Check sheet for the modelled part. Datum: model origin and axes. Units: mm. A direction names the side the tool comes from. Coordinates: 2 decimals unless noted, no trailing zeros. Write each loop counter-clockwise with the first axis right and the second up, starting at its lowest first coordinate (ties: lowest second). Pieces come first, ordered by that corner, then holes. Notation, with made-up numbers: (-37, 62) -> (-10, 62) arc R8 ccw to (-10, 71) -> close; hole circle Ø8 at (25.25, -26). An arc over 180 degrees is marked (long way). One line per item, written item: value. Start each with the question number.
1) Set-up check for faces 4 (the cylindrical face through (23.706, -22.68, 3.479)), 5 (the flat face through (13.895, 27, 1)), 6 (the flat face through (-25, 0, 1)), 7 (the flat face through (19, -25, 1)), 8 (the flat face through (-13.895, 27, 1)): record each of +Z, -Z, +X, -X, +Y, -Y from which the full face is reachable in a straight line by a thin tool's end or side.
2) Sectioned sample at B-B on y = 0. Enter the section's corners in (x, z), plus the area to 3 significant figures.
3) Scan lines: line 1 along Y through (x, z) = (0, 0.6); line 2 along Z through (x, y) = (-13, 29); line 3 along X through (y, z) = (23, 1.75). Record each from-to range of solid material in increasing order. Write a range as [from, to].
4) Gauge pin test, flat ends, axial feed: P1, Ø2, axis at x = -17.5, z = 0.5, coming from the +Y side; P2, Ø1, axis at x = 20, z = 1.5, coming from the -Y side; P3, Ø8, axis at x = -9, y = 23.5, coming from the +Z side. Record the tip position at first contact, or that the pin passes through.
5) Sectioned sample at C-C on z = 11.25. Enter the section's corners in (x, y), plus the area to 3 significant figures.
6) Sectioned sample at D-D on x = -16. Enter the section's corners in (y, z).
7) Sectioned sample at A-A on x = 0. Enter the section's corners in (y, z), plus the area to 3 significant figures.
8) Draft check along Y on faces 1 (the cylindrical face through (13.04, 31.6, 0.99)), 2 (the flat face through (-20, -25, 1)), 3 (the cylindrical face through (-21.836, -20.65, 2.535)). Enter one of: +Y half, -Y half, draft (parallel to the pull), parting line (faces both ways), or undercut.
```python
from build123d import *

# Parameters (mm, degrees)
F0_W      = 50
F0_H      = 50
F1_DEPTH  = 2
F2_R      = 2
F3_DEPTH  = 3
F4_R      = 1.5
F5_DEPTH  = 3
F7_DEPTH  = 2
F8_R      = 1.5
F9_DEPTH  = 25
F10_R     = 7.5
F11_DEPTH = 10
F12_R     = 5
F13_DEPTH = 10
F14_DEPTH = 7.7


# Not quite as in the source:
# - a pattern or mirror of a feature is missing from the dataset's text; its kind, count and spacing are read off the source's solid
# - a feature names something its author has since deleted; it is built from what else it names


with BuildPart() as f1:
    # F0 (on Top) → F1 (new body)
    with BuildSketch(Plane.XY):
        Rectangle(F0_W, F0_H)
    extrude(amount=F1_DEPTH)

    # F2 (on face) → F3 (join)
    with BuildSketch(Plane.XY.offset(2)):
        with Locations((-22.6419584364, -21.9144617685)):
            Circle(F2_R)
        with Locations((21.8580415636, -21.9144617685)):
            Circle(F2_R)
        with Locations((21.8580415636, 22.5855382315)):
            Circle(F2_R)
    f3 = extrude(amount=F3_DEPTH)

    # F3_copies: F3 across plane
    add(f3.mirror(Plane.ZX.offset(0.335538)))

    # F4 (on face) → F5 (cut)
    with BuildSketch(Plane.XY.offset(5)):
        with Locations((-22.6419584364, 22.5855382315)):
            Circle(F4_R)
        with Locations((21.8580415636, -21.9144617685)):
            Circle(F4_R)
        with Locations((21.8580415636, 22.5855382315)):
            Circle(F4_R)
        with Locations((-22.6419584364, -21.9144617685)):
            Circle(F4_R)
    extrude(amount=-F5_DEPTH, mode=Mode.SUBTRACT)

    # F6 (on Top) → F7 (join)
    with BuildSketch(Plane.XY):
        with BuildLine():
            ThreePointArc((13.8950906601, 29.5), (13.0164110037, 31.6213203436), (10.8950906601, 32.5))
            Line((10.8950906601, 32.5), (-10.8950906601, 32.5))
            ThreePointArc((-10.8950906601, 32.5), (-13.0164110037, 31.6213203436), (-13.8950906601, 29.5))
            Line((-13.8950906601, 29.5), (-13.8950906601, 25))
            Line((-13.8950906601, 25), (13.8950906601, 25))
            Line((13.8950906601, 25), (13.8950906601, 29.5))
        make_face()
        with BuildLine():
            Line((13.8950906601, -25), (-13.8950906601, -25))
            Line((-13.8950906601, -25), (-13.8950906601, -29.5))
            ThreePointArc((-13.8950906601, -29.5), (-13.0164110037, -31.6213203436), (-10.8950906601, -32.5))
            Line((-10.8950906601, -32.5), (10.8950906601, -32.5))
            ThreePointArc((10.8950906601, -32.5), (13.0164110037, -31.6213203436), (13.8950906601, -29.5))
            Line((13.8950906601, -29.5), (13.8950906601, -25))
        make_face()
    extrude(amount=F7_DEPTH)

    # F8 (on face) → F9 (cut)
    with BuildSketch(Plane.XY.offset(2)):
        with Locations((0, 29.5)):
            Circle(F8_R)
        with Locations((0, -29.5)):
            Circle(F8_R)
    extrude(amount=-F9_DEPTH, mode=Mode.SUBTRACT)

    # F10 (on face) → F11 (join)
    with BuildSketch(Plane.XY.offset(2)):
        Circle(F10_R)
    extrude(amount=F11_DEPTH)

    # F12 (on face) → F13 (cut)
    with BuildSketch(Plane.XY.offset(12)):
        Circle(F12_R)
    extrude(amount=-F13_DEPTH, mode=Mode.SUBTRACT)

    # F14 (cut): faces of the model
    f14_faces = [f1.faces().sort_by_distance(p)[0] for p in [
        (-22.6419584364, -21.9144617685, 2),
        (-22.6419584364, 22.5855382315, 2),
        (21.8580415636, 22.5855382315, 2),
        (21.8580415636, -21.9144617685, 2),
    ]]
    extrude(f14_faces, amount=-F14_DEPTH, mode=Mode.SUBTRACT)


solid = f1.part
```
Answers:
1. face 4: +Z
1. face 5: +Z, -Z, +X, +Y
1. face 6: +Z, -Z, -X, +Y, -Y
1. face 7: +Z, -Z, +X, -Y
1. face 8: +Z, -Z, -X, +Y
2. outline: (-25, 0) -> (25, 0) -> (25, 2) -> (7.5, 2) -> (7.5, 12) -> (5, 12) -> (5, 2) -> (-5, 2) -> (-5, 12) -> (-7.5, 12) -> (-7.5, 2) -> (-25, 2) -> close
2. area: 150 mm2
3. line 1: y = [-32.5, -31], [-28, 28], [31, 32.5]
3. line 2: z = [0, 2]
3. line 3: x = [-25, -24.08], [-21.2, 20.42], [23.3, 25]
4. P1: stops at y = 25
4. P2: stops at y = -25
4. P3: stops at z = 2
5. outline: circle Ø15 at (0, 0); hole circle Ø10 at (0, 0)
5. area: 98.2 mm2
6. outline: (-25, 0) -> (25, 0) -> (25, 2) -> (-25, 2) -> close
7. outline: (-32.5, 0) -> (-31, 0) -> (-31, 2) -> (-32.5, 2) -> close; (-28, 0) -> (28, 0) -> (28, 2) -> (7.5, 2) -> (7.5, 12) -> (5, 12) -> (5, 2) -> (-5, 2) -> (-5, 12) -> (-7.5, 12) -> (-7.5, 2) -> (-28, 2) -> close; (31, 0) -> (32.5, 0) -> (32.5, 2) -> (31, 2) -> close
7. area: 168 mm2
8. face 1: +Y half
8. face 2: -Y half
8. face 3: undercut
